Can you work these out from the model? Positions are in its coordinate system, mm. Give positions to 0.01 mm unless a question says otherwise; leave off trailing zeros. Order: outer loops, then holes, each group sorted by start corner. A loop starts at its lowest first (then second) coordinate and runs counter-clockwise, first axis right, second up. Notation, with made-up numbers: (-20.75, 53) - (7.25, 53) arc R34 cw to (7.25, 83) - close; hole circle Ø10 at (-17, 57.25). An arc over 180 degrees is marked (long way). Return JSON: item names as keys, results as strings.
Autodesk Inventor part; units mm, degrees
ref_plane "YZ Plane" through (0, 0, 0) normal (1, 0, 0) x (0, 1, 0)
ref_plane "XZ Plane" through (0, 0, 0) normal (0, 1, 0) x (-1, 0, 0)
ref_plane "XY Plane" through (0, 0, 0) normal (0, 0, 1) x (1, 0, 0)
sketch "Sketch1" plane through (0, 0, 0) normal (0, 0, 1) x (1, 0, 0)
  line L0 (19.05, -44.45) -> (-19.05, -44.45)
  line L1 (-19.05, -44.45) -> (-19.05, 44.45)
  line L2 (-19.05, 44.45) -> (19.05, 44.45)
  line L3 (19.05, 44.45) -> (19.05, -44.45)
  line L4 (19.05, -44.45) -> (-19.05, 44.45) construction
  line L5 (-19.05, -44.45) -> (19.05, 44.45) construction
  point P0 (0, 0)
  dimension "d0" = 38.1
  dimension "d1" = 88.9
extrude "Extrusion1" add sketch "Sketch1" along normal blind 254
sketch "Sketch2" plane through (0, 0, 254) normal (0, 0, 1) x (1, 0, 0)
  line L0 (-19.05, -44.45) -> (19.05, -44.45)
  line L1 (19.05, -44.45) -> (19.05, 44.45)
  line L2 (-3.175, -44.45) -> (19.05, -9.525)
  point P0 (0, 0)
  dimension "d7" = 22.225
  dimension "d8" = 34.925
extrude "Extrusion2" cut sketch "Sketch2" against normal blind 254
sketch "Sketch3" plane through (-19.05, -44.45, 0) normal (-1, 0, 0) x (0, 0, 1)
  line L0 (0, 0) -> (254, 0)
  arc A0 (177.8, 0) -> (76.2, 0) centre (127, -116.3974) ccw
  point P0 (0, 44.45)
  dimension "d11" = 76.2
  dimension "d12" = 76.2
  dimension "d13" = 127
extrude "Extrusion3" cut sketch "Sketch3" against normal blind 254
equation "\"d12\" = d11"
properties part number "ShooterFrontMount"
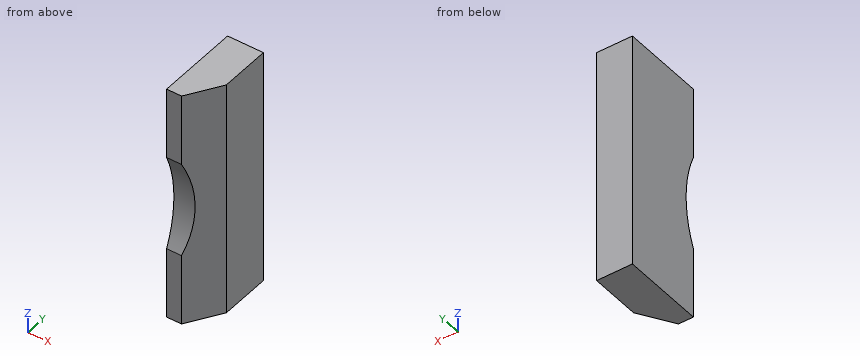
1. Suppose I cut it at C-C (z = 63.5). List the corners of the cut face in (x, y) for me (3 decimals).
Checks:
{"outline": "(-19.05, -44.45) - (-3.175, -44.45) - (19.05, -9.525) - (19.05, 44.45) - (-19.05, 44.45) - close"}
2. If I drill on L1, parallel to Y at x = 17.5, z = 48; L2, parallel to Y at x = 0, z = 97; L3, parallel to X at y = -37, z = 49, over which ranges is the centre line in solid material (lowest first)? Write a range as [from, to].
Checks:
{"L1": "[-11.96, 44.45]", "L2": "[-37.44, 44.45]", "L3": "[-19.05, 1.57]"}
3. Suppose I cut it at B-B (z = 127). List the corners of the cut face in (x, y) for me (3 decimals), plus the area to 3 significant figures.
Checks:
{"outline": "(-19.05, -33.847) - (3.572, -33.847) - (19.05, -9.525) - (19.05, 44.45) - (-19.05, 44.45) - close", "area": "2,790 mm^2"}
4. Suppose I cut it at A-A (x = -11). List the corners of the cut face in (y, z) for me, plus the area to 3 significant figures.
Checks:
{"outline": "(-44.45, 0) - (44.45, 0) - (44.45, 254) - (-44.45, 254) - (-44.45, 177.8) arc R127 cw to (-44.45, 76.2) - close", "area": "21,900 mm^2"}
5. Suppose I cut it at D-D (y = -12). List the corners of the cut face in (x, z) for me (3 decimals), plus the area to 3 significant figures.
Checks:
{"outline": "(-19.05, 0) - (17.475, 0) - (17.475, 254) - (-19.05, 254) - close", "area": "9,280 mm^2"}
